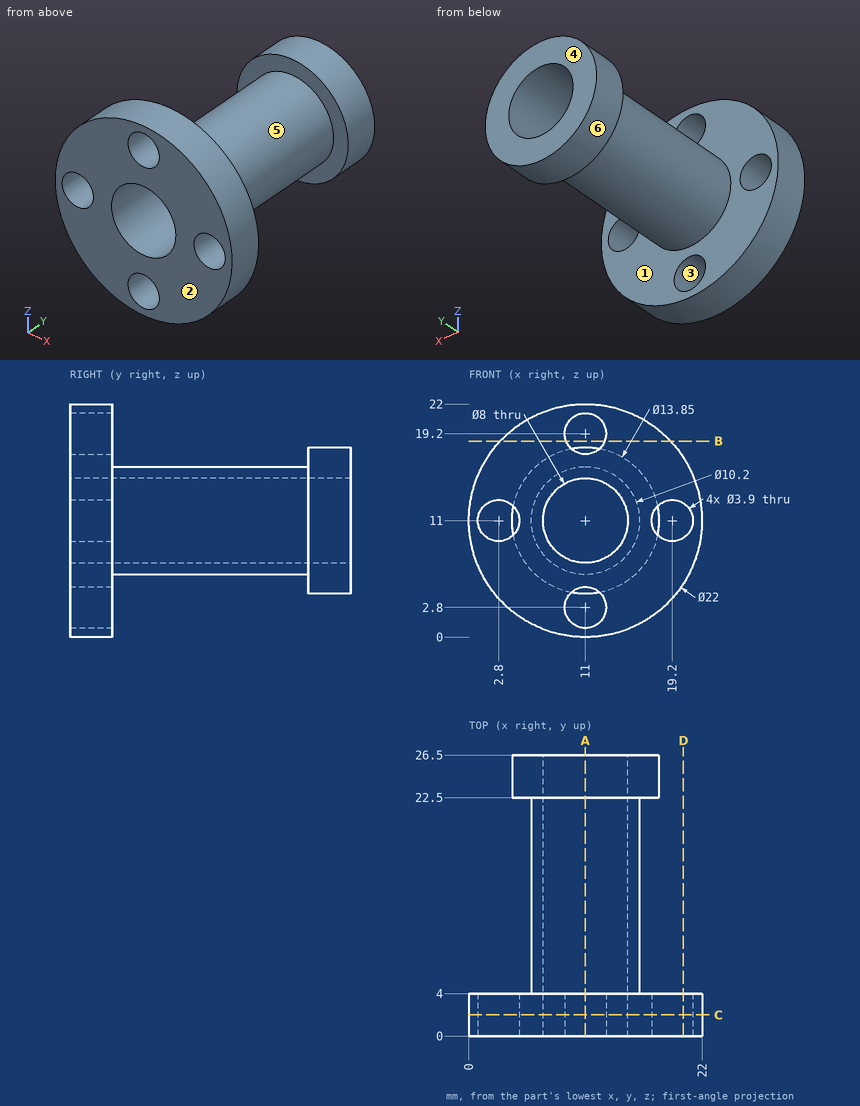
Study the drawing (mm; zero at the part's minimum x, y, z) and answer. A direction names the side the tool comes from. Give positions to 0.01 mm unless a question says otherwise; leave off trailing zeros. Order: outer loops, then holes, each group sorted by start corner. A loop starts at its lowest first (then second) coordinate and runs counter-clockwise, first axis right, second up. Notation, with made-up numbers: M 57.25,-23.75 L 71.25,-23.75 A17 ccw 71.25,-9.75 Z; hole C -9.5,-21.5 d8. An arc over 180 degrees is marked long. Put each result on its own line as item: value. Start each with the question number.
Item 1: The part is cut by section D-D, the plane x = 20.25. Determine the outline of the cut face in (y, z).
Item 2: The part is cut by section B-B, the plane z = 18.5. Determine the outline of the cut face in (x, y), and give its area (3 significant figures).
Item 3: The part is cut by section C-C, the plane y = 2. Determine the outline of the cut face in (x, z).
Item 4: Which of the six approach directions +Z, -Z, +X, -X, +Y, -Y give full straight-line access (tool end or side, diameter ignored) to the marked faces 1, 2 and 3?
Item 5: For a pull along Y with two mould halves and no side action, classify the marked faces 4, 5 and 6 as +Y half, -Y half, draft (parallel to the pull), parting line (faces both ways), or undercut.
Item 6: Flat-ended cylindrical pins translate along their axes: P1, Ø4, axis at x = 11, y = 9.5, coming from the -Z side; P2, Ø4, axis at x = 8, y = 7.5, coming from the +Z side; P3, Ø1.5, axis at y = 11, z = 10.5, coming from the -X side; P4, Ø1, axis at y = 5, z = 19.5, coming from the -X side. Find the tip coordinate at first contact, or state that the pin passes through.
Item 7: Find the intervals of material crossed by line 1 along X through (y, z) = (2.65, 11); line 2 along Y through (x, z) = (5.5, 11.25); line 3 along Y through (x, z) = (9, 18.75), in increasing order.
Item 8: The part is cut by section A-A, the plane x = 11. Determine the outline of the cut face in (y, z) (3 decimals), and give its area (3 significant figures).
Answer key:
1. outline: M 0,5.05 L 4,5.05 L 4,9.36 L 0,9.36 Z; M 0,12.64 L 4,12.64 L 4,16.95 L 0,16.95 Z
2. outline: M 2.95,0 L 9.18,0 L 9.18,4 L 2.95,4 Z; M 12.82,0 L 19.05,0 L 19.05,4 L 12.82,4 Z
2. area: 49.8 mm²
3. outline: C 11,11 d22; hole C 2.8,11 d3.9; hole C 11,11 d8; hole C 11,2.8 d3.9; hole C 11,19.2 d3.9; hole C 19.2,11 d3.9
4. face 1: none
4. face 2: +Z, -Z, +X, -X, -Y
4. face 3: -Y
5. face 4: +Y half
5. face 5: undercut
5. face 6: draft
6. P1: stops at z = 5.9
6. P2: stops at z = 16
6. P3: stops at x = 5.9
6. P4: passes through
7. line 1: x = 0 to 0.85, 4.75 to 7, 15 to 17.25, 21.15 to 22
7. line 2: y = 0 to 4, 22.5 to 26.5
7. line 3: y = 0 to 4
8. outline: M 0,0 L 4,0 L 4,0.85 L 0,0.85 Z; M 0,4.75 L 4,4.75 L 4,5.9 L 22.5,5.9 L 22.5,4.075 L 26.5,4.075 L 26.5,7 L 0,7 Z; M 0,15 L 26.5,15 L 26.5,17.925 L 22.5,17.925 L 22.5,16.1 L 4,16.1 L 4,17.25 L 0,17.25 Z; M 0,21.15 L 4,21.15 L 4,22 L 0,22 Z
8. area: 88.9 mm²
